Here's how the part is built. I have some questions about the finished solid (model axes, mm). Coordinates: 2 decimals unless noted, no trailing zeros. Order: outer loops, then holes, each group sorted by start corner. A loop starts at its lowest first (then second) coordinate and runs counter-clockwise, first axis right, second up. Notation, with made-up numbers: (-30.75, 38.5) - (16.25, 38.5) arc R18 cw to (16.25, 45.5) - close; hole circle Ø2 at (18, 25). An arc over 180 degrees is marked (long way). Use CSV: the item, a comma, the result in double quotes. Start each with the question number.
from build123d import *

# Parameters (mm, degrees)
F0_W     = 100.5
F0_H     = 82.5
F1_DEPTH = 2
F2_W     = 16.2
F2_H     = 16.2
F3_DEPTH = 25


with BuildPart() as f1:
    # F0 (on Front) → F1 (new body)
    with BuildSketch(Plane.XZ):
        with Locations((-67.112431, 2.068522)):
            Rectangle(F0_W, F0_H)
    extrude(amount=F1_DEPTH)

    # F2 (on Front) → F3 (cut)
    with BuildSketch(Plane.XZ):
        with Locations((-104.462431, 31.718522)):
            Rectangle(F2_W, F2_H)
        with Locations((-104.462431, 12.018522)):
            Rectangle(F2_W, F2_H)
        with Locations((-104.462431, -7.681478)):
            Rectangle(F2_W, F2_H)
        with Locations((-104.462431, -27.481478)):
            Rectangle(F2_W, F2_H)
        with Locations((-84.762431, 31.718522)):
            Rectangle(F2_W, F2_H)
        with Locations((-84.762431, 12.018522)):
            Rectangle(F2_W, F2_H)
        with Locations((-84.762431, -7.681478)):
            Rectangle(F2_W, F2_H)
        with Locations((-65.062431, 31.718522)):
            Rectangle(F2_W, F2_H)
        with Locations((-65.062431, 12.018522)):
            Rectangle(F2_W, F2_H)
        with Locations((-65.062431, -7.681478)):
            Rectangle(F2_W, F2_H)
        with Locations((-45.362431, 31.718522)):
            Rectangle(F2_W, F2_H)
        with Locations((-45.362431, 12.018522)):
            Rectangle(F2_W, F2_H)
        with Locations((-45.362431, -7.681478)):
            Rectangle(F2_W, F2_H)
        with Locations((-75.662431, -27.079934)):
            Rectangle(F2_W, F2_H)
        with Locations((-35.762431, -27.481478)):
            Rectangle(F2_W, F2_H)
        with Locations((-25.662431, -7.731478)):
            Rectangle(F2_W, F2_H)
        with Locations((-25.662431, 22.468522)):
            Rectangle(F2_W, F2_H)
    extrude(amount=F3_DEPTH, mode=Mode.SUBTRACT)


solid = f1.part
Item 1: Suppose I cut it at D-D on y = -0.65. State how many separate pieces and enclosed holes the cut face has, then the cut area to 3 significant figures.
Item 2: Suppose I cut it at C-C on x = -35. Write out the boundary of the cut face in (y, z).
Item 3: Please list where these lines run through material, in increasing order: line 1 along X through (y, z) = (-1.8, -28.5); line 2 along X through (y, z) = (-1.4, -4); line 3 along Z through (x, y) = (-72.5, -0.45). Write a range as from..to.
Item 4: We'd pull the mould along Z, two halves only. Please class faces 1 (the flat face through (-68, -1, -39.181)), 2 (the flat face through (-76.662, -1, 32)): released by +Z, released by -Z, zero draft, split by the parting line, or undercut.
Item 5: Suppose I cut it at B-B on z = 32.5. Write out the boundary of the cut face in (x, y).
Item 6: Suppose I cut it at A-A on x = -86. Write out the boundary of the cut face in (y, z).
Here are the results:
1,separate pieces,"1"
1,enclosed holes,"17"
1,area,"3,830 mm^2"
2,outline,"(-2, -39.18) - (0, -39.18) - (0, -35.58) - (-2, -35.58) - close; (-2, -19.38) - (0, -19.38) - (0, 43.32) - (-2, 43.32) - close"
3,line 1,"-117.36..-112.56, -96.36..-83.76, -67.56..-43.86, -27.66..-16.86"
3,line 2,"-117.36..-112.56, -96.36..-92.86, -76.66..-73.16, -56.96..-53.46, -37.26..-33.76, -17.56..-16.86"
3,line 3,"-39.18..-35.18, -18.98..-15.78, 0.42..3.92, 20.12..23.62, 39.82..43.32"
4,face 1,"released by -Z"
4,face 2,"undercut"
5,outline,"(-117.36, -2) - (-112.56, -2) - (-112.56, 0) - (-117.36, 0) - close; (-96.36, -2) - (-92.86, -2) - (-92.86, 0) - (-96.36, 0) - close; (-76.66, -2) - (-73.16, -2) - (-73.16, 0) - (-76.66, 0) - close; (-56.96, -2) - (-53.46, -2) - (-53.46, 0) - (-56.96, 0) - close; (-37.26, -2) - (-16.86, -2) - (-16.86, 0) - (-37.26, 0) - close"
6,outline,"(-2, -39.18) - (0, -39.18) - (0, -15.78) - (-2, -15.78) - close; (-2, 0.42) - (0, 0.42) - (0, 3.92) - (-2, 3.92) - close; (-2, 20.12) - (0, 20.12) - (0, 23.62) - (-2, 23.62) - close; (-2, 39.82) - (0, 39.82) - (0, 43.32) - (-2, 43.32) - close"
